Design review of the part built by this model. Coordinates are the model's own, in mm. Coordinates: 2 decimals unless noted, no trailing zeros. Loops run counter-clockwise (first coordinate to the right, second up) from the corner with the lowest first, then second, coordinate; pieces in that order, holes last.
Q1. Add section B-B on x = 12. Give the boundary of the cut face in (y, z).
Q2. Add section D-D on y = 22. Give the boundary of the cut face in (x, z).
Q3. Draft analysis for pull direction X (two halves, no side actions). For faces 1 (the face through (8.9, 15.07, 2.46)), 2 (the face through (-12, 20, 5.5)), 3 (the face through (-21.625, 16.581, 2.465)), state which applies: released by +X, released by -X, zero draft, split by the parting line, or undercut.
Q4. Add section C-C on z = 3.9. Give the boundary of the cut face in (x, y), and give its area (3 significant figures).
Q5. For P1, Ø10, axis at x = 9.5, y = -1.5, coming from the +Z side; P2, Ø3, axis at x = -3, z = 4, coming from the +Y side; P3, Ø2, axis at y = -11.5, z = 4.5, coming from the -X side, all flat-tipped, find the tip position at first contact; note any pin that passes through.
Q6. Add section A-A on y = -2.5. Give the boundary of the cut face in (x, z).
Q7. Wall thickness on probe 1 along Z at (x, y) = (16, 20); probe 2 along Y at (x, z) = (15, 2.3); probe 3 along Y at (x, z) = (16.5, 0.6): over which ranges is each line inside the solid? List them lowest first.
Autodesk Inventor part; units mm, degrees
ref_plane "YZ Plane" through (0, 0, 0) normal (1, 0, 0) x (0, 1, 0)
ref_plane "XZ Plane" through (0, 0, 0) normal (0, 1, 0) x (-1, 0, 0)
ref_plane "XY Plane" through (0, 0, 0) normal (0, 0, 1) x (1, 0, 0)
sketch "Esquisse1" plane through (0, 0, 0) normal (0, 0, 1) x (1, 0, 0)
  circle A0 centre (0, 0) radius 27
  circle A1 centre (-1.666702, -13.02482) radius 15.430073
  circle A2 centre (14.698986, 3.590179) radius 12.859707
  circle A3 centre (0, 0) radius 27.25
  circle A4 centre (0.777883, 3.425174) radius 0.684809
  circle A5 centre (-18.340493, -16.491398) radius 0.684809
  circle A6 centre (-11.511215, 19.899288) radius 1.369619
  circle A7 centre (18.687299, 17.311193) radius 0.684809
  point P0 (1.940785, 1.977619)
  point P1 (23.885419, 12.589152)
  point P2 (-12.669004, -23.843161)
  dimension "d0" = 54
  dimension "d6" = 54.5
  dimension "d9" = 1.36962
sketch "Esquisse1 outline for Cadran" plane through (0, 0, 0) normal (0, 0, 1) x (1, 0, 0)
  circle A0 centre (0, 0) radius 27.25
  arc A1 (23.885419, 12.589152) -> (-12.669004, -23.843161) centre (0, 0) cw
  arc A2 (1.940785, 1.977619) -> (23.885419, 12.589152) centre (14.698986, 3.590179) cw
  arc A3 (-12.669004, -23.843161) -> (1.940785, 1.977619) centre (-1.666702, -13.02482) cw
extrude "Cadran" add sketch "Esquisse1 outline for Cadran" along normal blind 5
sketch "Esquisse4" plane through (0, 0, 5) normal (0, 0, 1) x (1, 0, 0)
  circle A0 centre (-11.643189, 19.963438) radius 1.192314
  circle A1 centre (0.805137, 3.454442) radius 0.685
  circle A2 centre (-18.727601, -16.711919) radius 0.685
  circle A3 centre (18.709962, 17.292624) radius 0.685
  point P0 (0, 0)
  dimension "d10" = 1.37
extrude "Emplacements Vis" add sketch "Esquisse4" along normal blind 0.5
fillet "Congé1" radius 0.5 1 edges at (18.025, 17.2926, 5.5)
fillet "Congé2" radius 0.5 1 edges at (0.1201, 3.4544, 5.5)
fillet "Congé3" radius 0.5 1 edges at (-12.8355, 19.9634, 5.5)
fillet "Congé4" radius 0.5 1 edges at (-19.4126, -16.7119, 5.5)
properties part number "Candran face cache"
Entries:
1. outline: (-24.47, 0) - (-24.19, 0) - (-24.19, 5) - (-24.47, 5) - close; (16.16, 0) - (24.47, 0) - (24.47, 5) - (16.16, 5) - close
2. outline: (-16.08, 0) - (16.08, 0) - (16.08, 5) - (-16.08, 5) - close
3. face 1: undercut
3. face 2: zero draft
3. face 3: split by the parting line
4. outline: circle Ø54.5 at (0, 0); hole (-12.67, -23.84) arc R27 ccw to (23.89, 12.59) arc R12.86 ccw to (1.94, 1.98) arc R15.43 ccw to start
4. area: 1,000 mm2
5. P1: passes through
5. P2: stops at y = 27.21
5. P3: stops at x = -25.15
6. outline: (-27.14, 0) - (-12.95, 0) - (-12.95, 5) - (-27.14, 5) - close; (26.88, 0) - (27.14, 0) - (27.14, 5) - (26.88, 5) - close
7. probe 1: z = 0 to 5
7. probe 2: y = -22.75 to -22.45, 16.45 to 22.75
7. probe 3: y = -21.69 to -21.37, 16.32 to 21.69
